```python
from build123d import *

# Parameters (mm, degrees)
F0_R         = 1.6
F1_DEPTH     = 5
F2_DEPTH     = 1
F3_R         = 15.5
F3_R_2       = 14
F4_DEPTH     = 11.5
F5_SIZE2     = 1.5
F5_SIZE      = 1
F8_T4_ANGLE  = 185.4300536725
F8_S5_R      = 22.5
F8_T6_DEPTH  = 9
F8_T10_ANGLE = 185.4300536725
F8_S11_R     = 22.5
F8_T12_DEPTH = 9
F9_R         = 5
F10_DEPTH    = 3
F11_R        = 3.25
F12_DEPTH    = 5


# Not quite as in the source:
# - a fillet or chamfer that OpenCascade refuses, or shapes differently, is made with other operations: its cross-section is extruded or revolved along the edge and cut away or added
# - a feature of the source that left no trace in its solid (it failed there, or was rolled back) is left out


with BuildPart() as f1:
    # F0 (on Top) → F1 (new body)
    with BuildSketch(Plane.XY):
        with BuildLine():
            ThreePointArc((-22.1862745098, -3.7442253372), (-22.5, 0), (-22.1862745098, 3.7442253372))
            ThreePointArc((-22.1862745098, 3.7442253372), (-30.5, 0), (-22.1862745098, -3.7442253372))
        make_face()
        with Locations((-25.5, 0)):
            Circle(F0_R, mode=Mode.SUBTRACT)
        with BuildLine():
            ThreePointArc((-20.5, 0), (-20.9410183456, 2.0532136456), (-22.1862745098, 3.7442253372))
            ThreePointArc((-22.1862745098, 3.7442253372), (-22.5, 0), (-22.1862745098, -3.7442253372))
            ThreePointArc((-22.1862745098, -3.7442253372), (-20.9410183456, -2.0532136456), (-20.5, 0))
        make_face()
    extrude(amount=F1_DEPTH)



with BuildPart() as f1b:
    # F0 (on Top) → F1, piece 2 (new body)
    with BuildSketch(Plane.XY):
        with BuildLine():
            ThreePointArc((22.1862745098, 3.7442253372), (22.4214314493, 1.8786728733), (22.5, 0))
            ThreePointArc((22.5, 0), (22.4214314493, -1.8786728733), (22.1862745098, -3.7442253372))
            ThreePointArc((22.1862745098, -3.7442253372), (27.5532136456, -4.5589816544), (30.5, 0))
            ThreePointArc((30.5, 0), (27.5532136456, 4.5589816544), (22.1862745098, 3.7442253372))
        make_face()
        with Locations((25.5, 0)):
            Circle(F0_R, mode=Mode.SUBTRACT)
        with BuildLine():
            ThreePointArc((22.1862745098, -3.7442253372), (22.4214314493, -1.8786728733), (22.5, 0))
            ThreePointArc((22.5, 0), (22.4214314493, 1.8786728733), (22.1862745098, 3.7442253372))
            ThreePointArc((22.1862745098, 3.7442253372), (20.5, 0), (22.1862745098, -3.7442253372))
        make_face()
    extrude(amount=F1_DEPTH)


with BuildPart() as f1_1:
    add(f1.part)

    add(f1b.part)  # F2 merges F1b
    # F0 (on Top) → F2 (join)
    with BuildSketch(Plane.XY):
        with BuildLine():
            ThreePointArc((22.1862745098, -3.7442253372), (20.5, 0), (22.1862745098, 3.7442253372))
            ThreePointArc((22.1862745098, 3.7442253372), (0, 22.5), (-22.1862745098, 3.7442253372))
            ThreePointArc((-22.1862745098, 3.7442253372), (-20.9410183456, 2.0532136456), (-20.5, 0))
            ThreePointArc((-20.5, 0), (-20.9410183456, -2.0532136456), (-22.1862745098, -3.7442253372))
            ThreePointArc((-22.1862745098, -3.7442253372), (0, -22.5), (22.1862745098, -3.7442253372))
        make_face()
    extrude(amount=F2_DEPTH)

    # F3 (on face) → F4 (join)
    with BuildSketch(Plane.XY.offset(1)):
        Circle(F3_R)
        Circle(F3_R_2, mode=Mode.SUBTRACT)
    extrude(amount=F4_DEPTH)

    # F5
    f5_edges = [f1_1.edges().sort_by_distance(p)[0] for p in [
        (-15.5, 0, 12.5),
    ]]
    f5_side = f1_1.faces().sort_by_distance((-15.061594, 0, 12.5))[0]
    chamfer(f5_edges, length=F5_SIZE, length2=F5_SIZE2, reference=f5_side)

    # F8: chamfer of 1.5 on 2 edges, made by hand


with BuildPart() as f8_tool2:
    # F8_s3 → F8_t4 (revolve)
    with BuildSketch(Plane(origin=(25.4427839223, 1.2065389767, 0), x_dir=(0, 0, 1), z_dir=(0.9988774861, 0.0473684257, 0))):
        Polygon((1, 7.7078948555), (2.5, 6.2078948555), (1, 6.2078948555), align=None)
    revolve(axis=Axis((25.5, 0, 1), (0, 0, -1)), revolution_arc=F8_T4_ANGLE)

    # F8_s5 → F8_t6 (intersect, symmetric)
    with BuildSketch(Plane.XY.offset(1.8)):
        Circle(F8_S5_R)
    extrude(amount=F8_T6_DEPTH, both=True, mode=Mode.INTERSECT)


with BuildPart() as f1_2:
    add(f1_1.part)

    # F8_t1: union F8_tool2
    add(f8_tool2.part)


with BuildPart() as f8_tool8:
    # F8_s9 → F8_t10 (revolve)
    with BuildSketch(Plane(origin=(-25.4427839223, 1.2065389767, 0), x_dir=(0, 0, 1), z_dir=(-0.9988774861, 0.0473684257, 0))):
        Polygon((1, -7.7078948555), (2.5, -6.2078948555), (1, -6.2078948555), align=None)
    revolve(axis=Axis((-25.5, 0, 1), (0, 0, 1)), revolution_arc=F8_T10_ANGLE)

    # F8_s11 → F8_t12 (intersect, symmetric)
    with BuildSketch(Plane.XY.offset(1.7)):
        Circle(F8_S11_R)
    extrude(amount=F8_T12_DEPTH, both=True, mode=Mode.INTERSECT)


with BuildPart() as f1_3:
    add(f1_2.part)

    # F8_t7: union F8_tool8
    add(f8_tool8.part)

    # F9 (on face) → F10 (join)
    with BuildSketch(Plane.XY.offset(1)):
        Circle(F9_R)
    extrude(amount=F10_DEPTH)

    # F11 (on face) → F12 (cut)
    with BuildSketch(Plane.XY.offset(4)):
        Circle(F11_R)
    extrude(amount=-F12_DEPTH, mode=Mode.SUBTRACT)


solid = f1_3.part
```
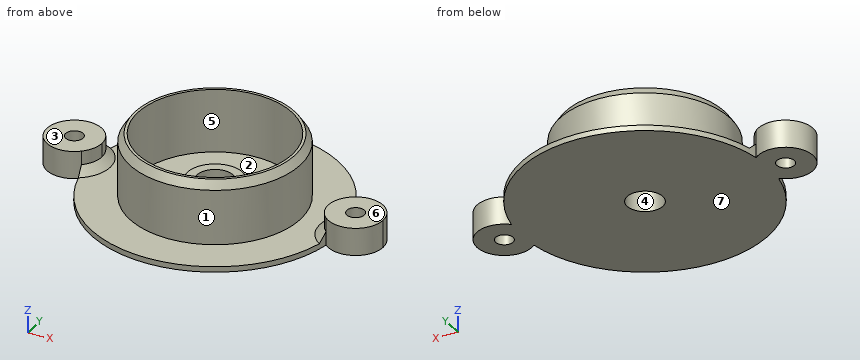
Can you work these out from the model? Positions are in its coordinate system, mm. Face numbers are marked on the shaded views. A direction names the side the tool comes from. Round coordinates to 2 decimals unless told otherwise and drop trailing zeros. Loops run counter-clockwise (first coordinate to the right, second up) from the corner with the lowest first, then second, coordinate; pieces in that order, holes last. Notation, with made-up numbers: M 14.5,77.25 L 38.5,77.25 A21 ccw 38.5,115.25 Z; hole C 47.5,83.5 d1. An arc over 180 degrees is marked long. Answer as a JSON object with one key per item and string values. Group by question number.
Q1. Please list where these lines run through material, in increasing order: L1, parallel to Y at x = 0, z = 3.15; L2, parallel to Y at x = 0, z = 5.5; L3, parallel to Y at x = 25.5, z = 2.3.
Q2. Imagine slicing it at A-A, the plane x = 25.5. Please give me the cut outline in (y, z).
Q3. Will these pins go through, and if not, where does the flat tip stop? pin 1 (5 mm diameter, centred on x = 2, y = 0, fed in from +Z); pin 2 (4 mm diameter, centred on x = 3.5, z = 10, fed in from -Y); pin 3 (4 mm diameter, centred on y = 3.5, z = 8, fed in from -X); pin 4 (1 mm diameter, centred on y = 17.5, z = 3, fed in from -X).
Q4. Imagine slicing it at B-B, the plane z = 7.5. Please give me the cut outline in (x, y), then the cut area to 3 significant figures.
Q5. Imagine slicing it at C-C, the plane x = 0. Please give me the cut outline in (y, z), then the cut area to 3 significant figures.
Q6. We'd pull the mould along Y, two halves only. Please class the marked faces 1, 2, 3 and 4: +Y half, -Y half, draft (parallel to the pull), parting line (faces both ways), or undercut.
Q7. On a 3-axis mill with a long thin cutter (end or side, diameter ignored), from which of +Z, -Z, +X, -X, +Y, -Y can I reach the whole of each face in a straight line? I mean the marked faces 5, 6 and 7. Say none if no direction works.
Findings:
{
 "1": {"L1": "y = -15.5 to -14, -5 to -3.25, 3.25 to 5, 14 to 15.5", "L2": "y = -15.5 to -14, 14 to 15.5", "L3": "y = -5 to -1.6, 1.6 to 5"},
 "2": {"outline": "M -5,0 L -1.6,0 L -1.6,5 L -5,5 Z; M 1.6,0 L 5,0 L 5,5 L 1.6,5 Z"},
 "3": {"pin 1": "stops at z = 4", "pin 2": "stops at y = -15.43", "pin 3": "stops at x = -15.43", "pin 4": "passes through"},
 "4": {"outline": "C 0,0 d31; hole C 0,0 d28", "area": "139 mm2"},
 "5": {"outline": "M -22.5,0 L -3.25,0 L -3.25,4 L -5,4 L -5,1 L -14,1 L -14,12.5 L -14.5,12.5 L -15.5,11 L -15.5,1 L -22.5,1 Z; M 3.25,0 L 22.5,0 L 22.5,1 L 15.5,1 L 15.5,11 L 14.5,12.5 L 14,12.5 L 14,1 L 5,1 L 5,4 L 3.25,4 Z", "area": "82.0 mm2"},
 "6": {"face 1": "parting line", "face 2": "undercut", "face 3": "draft", "face 4": "undercut"},
 "7": {"face 5": "+Z", "face 6": "+Z, +X, +Y, -Y", "face 7": "-Z, +X, -X, +Y, -Y"}
}
